Build history of the part. All positions in model axes, mm. Round coordinates to 2 decimals unless told otherwise and drop trailing zeros. Write each loop counter-clockwise with the first axis right and the second up, starting at its lowest first coordinate (ties: lowest second). Pieces come first, ordered by that corner, then holes. Notation, with made-up numbers: M 28.25,-34.5 L 36.25,-34.5 A14 cw 36.25,-17.5 Z; hole C -9.5,-12 d4. An arc over 180 degrees is marked long. One line per item, written item: value. Start each with the question number.
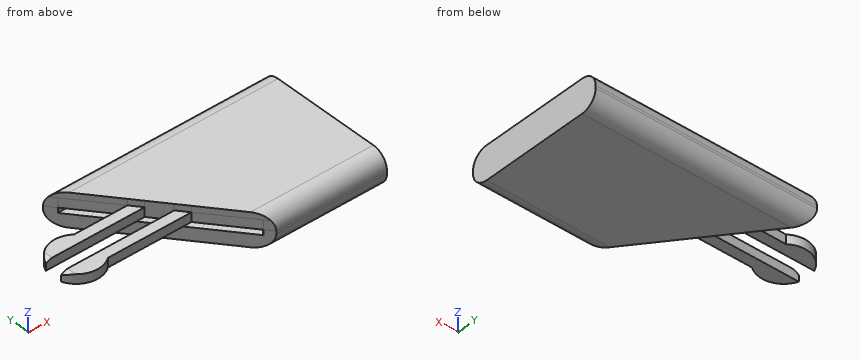
```python
from build123d import *

# Parameters (mm, degrees)
F2_DEPTH  = 3.5
F4_DEPTH  = 1
F6_DEPTH  = 1.8
F8_DEPTH  = 1.2
F9_R      = 3
F11_DEPTH = 17.1864665007


with BuildPart() as f2:
    # F1 (on Top) → F2 (new body)
    with BuildSketch(Plane.XY):
        Polygon((48.5598316574, 13.5), (5.4801683426, 13.5), (27.0198316574, -13.5), align=None)
        Polygon((48.5598316574, 13.5), (27.0198316574, -13.5), (48.5598316574, -13.5), align=None)
    extrude(amount=-F2_DEPTH)

    # F3 (on Top) → F4 (cut)
    with BuildSketch(Plane.XY):
        Polygon((44.7943471372, 11.7882982132), (6.8457046456, 11.7882982132), (25.8198775993, -11.9958558036), align=None)
    extrude(amount=-F4_DEPTH, mode=Mode.SUBTRACT)

    # F5 (on face) → F6 (join)
    with BuildSketch(Plane.XY):
        with BuildLine():
            ThreePointArc((2.8793278964, 3.7278809202), (3.7658696299, 2.8294612951), (4.3820146982, 1.7278809202))
            Line((4.3820146982, 1.7278809202), (14.8715565456, 1.7278809202))
            Line((14.8715565456, 1.7278809202), (17.594606702, -1.6854665007))
            Line((17.594606702, -1.6854665007), (4.3985029231, -1.6854665007))
            ThreePointArc((4.3985029231, -1.6854665007), (3.7999051439, -2.783585132), (2.9334215452, -3.6854665007))
            Line((2.9334215452, -3.6854665007), (19.1901373179, -3.6854665007))
            Line((19.1901373179, -3.6854665007), (25.8198775993, -11.9958558036))
            Line((25.8198775993, -11.9958558036), (44.7943471372, 11.7882982132))
            Line((44.7943471372, 11.7882982132), (6.8457046456, 11.7882982132))
            Line((6.8457046456, 11.7882982132), (13.2760259297, 3.7278809202))
            Line((13.2760259297, 3.7278809202), (2.8793278964, 3.7278809202))
        make_face()
        Polygon((5.4801683426, 13.5), (6.8457046456, 11.7882982132), (44.7943471372, 11.7882982132), (25.8198775993, -11.9958558036), (27.0198316574, -13.5), (48.5598316574, 13.5), align=None)
        with BuildLine():
            Line((-4.3820146982, 1.7278809202), (4.3820146982, 1.7278809202))
            ThreePointArc((4.3820146982, 1.7278809202), (3.7658696299, 2.8294612951), (2.8793278964, 3.7278809202))
            ThreePointArc((2.8793278964, 3.7278809202), (-1.2508065023, 4.5412672663), (-4.3820146982, 1.7278809202))
        make_face()
        with BuildLine():
            ThreePointArc((2.9334215452, -3.6854665007), (3.7999051439, -2.783585132), (4.3985029231, -1.6854665007))
            Line((4.3985029231, -1.6854665007), (-4.3985029231, -1.6854665007))
            ThreePointArc((-4.3985029231, -1.6854665007), (-1.2396031062, -4.5443381728), (2.9334215452, -3.6854665007))
        make_face()
        Polygon((48.5598316574, 13.5), (27.0198316574, -13.5), (48.5598316574, -13.5), align=None)
    extrude(amount=F6_DEPTH)

    # F7 (on face) → F8 (join)
    with BuildSketch(Plane.XY.offset(1.8)):
        Polygon((48.5598316574, 13.5), (5.4801683426, 13.5), (13.2760259297, 3.7278809202), (14.8715565456, 1.7278809202), (17.594606702, -1.6854665007), (19.1901373179, -3.6854665007), (27.0198316574, -13.5), (48.5598316574, -13.5), align=None)
    extrude(amount=F8_DEPTH)

    # F9
    f9_edges = [f2.edges().sort_by_distance(p)[0] for p in [
        (27.02, 13.5, 3),
        (27.02, 13.5, -3.5),
        (37.789832, -13.5, 3),
        (37.789832, -13.5, -3.5),
    ]]
    fillet(f9_edges, radius=F9_R)

    # F10 (on face) → F11 (cut, through all)
    with BuildSketch(Plane.XZ.offset(3.6854665007)):
        with BuildLine():
            ThreePointArc((-4.430251196, 1.1966986349), (-3.7397455906, 1.6462971281), (-2.9335320779, 1.8164634239))
            Line((-2.9335320779, 1.8164634239), (-4.430251196, 1.8164634239))
            Line((-4.430251196, 1.8164634239), (-4.430251196, 1.1966986349))
        make_face()
    extrude(amount=-F11_DEPTH, mode=Mode.SUBTRACT)


solid = f2.part
```
Item 1: Cut at A-A, the plane x = 33. Write the cut outline in (y, z).
Item 2: Cut at B-B, the plane x = 14. Write the cut outline in (y, z), plus the area to 3 significant figures.
Item 3: Drill centre lines: line 1 (Z direction, x = 43, y = 10.75); line 2 (Y direction, x = 13, z = 0.25); line 3 (Y direction, x = 3.5, z = 1.75). Where is each one in solid material? Low to high.
Item 4: Cut at C-C, the plane y = -11.5. Write the cut outline in (x, z), plus the area to 3 significant figures.
Item 5: Drop flat-ended pins along their axis: pin 1 (0.5 mm diameter, centred on x = 9.5, z = 0.5, fed in from -Y); pin 2 (1 mm diameter, centred on x = 32, z = 1, fed in from -Y); pin 3 (3.5 mm diameter, centred on x = 1.5, y = 3, fed in from +Z). Give the stop position or say it passes through.
Item 6: Cut at D-D, the plane z = -2. Write the cut outline in (x, y).
Computed values:
1. outline: M -13.5,-0.5 A3 ccw -10.5,-3.5 L 10.5,-3.5 A3 ccw 13.5,-0.5 L 13.5,0 A3 ccw 10.5,3 L -10.5,3 A3 ccw -13.5,0 Z; hole M -3,-1 L 11.79,-1 L 11.79,0 L -3,0 Z
2. outline: M -3.69,0 L -1.69,0 L -1.69,1.8 L -3.69,1.8 Z; M 1.73,0 L 11.79,0 L 11.79,-1 L 2.82,-1 L 2.82,-3.5 L 10.5,-3.5 A3 ccw 13.5,-0.5 L 13.5,0 A3 ccw 10.5,3 L 2.82,3 L 2.82,1.8 L 1.73,1.8 Z
2. area: 62.2 mm2
3. line 1: z = -3.49 to -1, 0 to 2.99
3. line 2: y = -3.69 to -1.69, 1.73 to 3.73, 4.07 to 13.49
3. line 3: y = -3.69 to -1.69, 1.73 to 3.73
4. outline: M 25.42,-3.33 L 48.56,-3.33 L 48.56,2.83 L 25.42,2.83 L 25.42,0 L 26.22,0 L 26.22,-1 L 25.42,-1 Z
4. area: 142 mm2
5. pin 1: stops at y = -3.69
5. pin 2: stops at y = -13.46
5. pin 3: stops at z = 1.8
6. outline: M 5.8,13.1 L 26.7,-13.1 L 48.56,-13.1 L 48.56,13.1 Z
